The listing builds one solid part. Answer for the finished solid, in the listing's coordinates (mm). Round coordinates to 2 decimals unless told otherwise and drop trailing zeros. Write each loop counter-clockwise with the first axis right and the second up, starting at its lowest first coordinate (ties: lowest second). Pieces come first, ordered by that corner, then holes. Notation, with made-up numbers: (6.5, 74.25) - (23.5, 74.25) arc R23 ccw to (23.5, 95.25) - close; hole circle Ø7 at (59, 52.5). An arc over 180 degrees is marked (long way). Return JSON: item names as keys, results as strings. Group by question number.
(1) Section C-C, the plane x = -87 is taken. Write down the section's boundary in (y, z), then the cut area to 3 significant figures.
(2) Section B-B, the plane z = 1.1 is taken. Give the number of separate pieces and of enclosed holes in the cut face, then the cut area to 3 significant figures.
(3) Section A-A, the plane y = 2 is taken. Write down the section's boundary in (x, z).
(4) Find the intervals of material crossed by line 1 along X through (y, z) = (-32.5, 2.25); line 2 along X through (y, z) = (-71.5, 1.55); line 3 along X through (y, z) = (-113.5, 4.65), in increasing order. Write a range as [from, to].
(5) Each of these flat-tipped pins is pushed along its axis until it touches: pin 1 (1 mm diameter, centred on y = -82.5, z = 2, fed in from -X); pin 2 (6 mm diameter, centred on x = 94.92, y = -69.92, fed in from -Z); pin 3 (2.5 mm diameter, centred on y = -109, z = 2, fed in from +X). Where does it stop, or does it pass through?
```python
from build123d import *

# Parameters (mm, degrees)
F0_W      = 220
F0_H      = 170
F0_W_2    = 200
F0_H_2    = 150
F1_DEPTH  = 5
F2_W      = 5.5
F2_H      = 21
F3_DEPTH  = 25
F4_W      = 12
F4_H      = 5
F5_DEPTH  = 45
F6_R      = 2.2
F7_DEPTH  = 25
F8_R      = 5.99999
F9_R      = 6
F10_R     = 4
F11_DEPTH = 2.5
F13_R     = 5
F15_DEPTH = 3
F12_R     = 2.5
F16_DEPTH = 3


# Not quite as in the source:
# - a fillet or chamfer is up to 0.001 mm smaller than in the source, because OpenCascade refuses the exact size


with BuildPart() as f1:
    # F0 (on Top) → F1 (new body)
    with BuildSketch(Plane.XY):
        Rectangle(F0_W, F0_H)
        Rectangle(F0_W_2, F0_H_2, mode=Mode.SUBTRACT)
        Rectangle(F0_W_2, F0_H_2)
    extrude(amount=F1_DEPTH)

    # F2 (on face) → F3 (cut)
    with BuildSketch(Plane.XY.offset(5)):
        with Locations((-105, 60)):
            Rectangle(F2_W, F2_H)
        with Locations((-105, 10)):
            Rectangle(F2_W, F2_H)
        with Locations((-105, -40)):
            Rectangle(F2_W, F2_H)
        with Locations((105, 60)):
            Rectangle(F2_W, F2_H)
        with Locations((105, 10)):
            Rectangle(F2_W, F2_H)
        with Locations((105, -40)):
            Rectangle(F2_W, F2_H)
    extrude(amount=-F3_DEPTH, mode=Mode.SUBTRACT)

    # F4 (on face) → F5 (join)
    with BuildSketch(Plane.XZ.offset(85)):
        with Locations((59, 2.5)):
            Rectangle(F4_W, F4_H)
        with Locations((-59, 2.5)):
            Rectangle(F4_W, F4_H)
    extrude(amount=F5_DEPTH)

    # F6 (on face) → F7 (cut)
    with BuildSketch(Plane.XY.offset(5)):
        with Locations((-59, -74.3)):
            Circle(F6_R)
        with Locations((-59, -124)):
            Circle(F6_R)
        with Locations((59, -74.3)):
            Circle(F6_R)
        with Locations((59, -124)):
            Circle(F6_R)
    extrude(amount=-F7_DEPTH, mode=Mode.SUBTRACT)

    # F8 (radius 6 in the source; OpenCascade refuses exactly that, so slightly less here)
    f8_edges = [f1.edges().sort_by_distance(p)[0] for p in [
        (-65, -130, 2.5),
        (-53, -130, 2.5),
        (53, -130, 2.5),
        (65, -130, 2.5),
    ]]
    fillet(f8_edges, radius=F8_R)

    # F9
    f9_edges = [f1.edges().sort_by_distance(p)[0] for p in [
        (-65, -85, 2.5),
        (-53, -85, 2.5),
        (53, -85, 2.5),
        (65, -85, 2.5),
    ]]
    fillet(f9_edges, radius=F9_R)

    # F10 (on face) → F11 (cut)
    with BuildSketch(Plane.XY.offset(5)):
        with Locations((-59, -124)):
            Circle(F10_R)
        with Locations((-59, -74.3)):
            Circle(F10_R)
        with Locations((59, -74.3)):
            Circle(F10_R)
        with Locations((59, -124)):
            Circle(F10_R)
    extrude(amount=-F11_DEPTH, mode=Mode.SUBTRACT)

    # F13
    f13_edges = [f1.edges().sort_by_distance(p)[0] for p in [
        (-110, -85, 2.5),
        (110, -85, 2.5),
        (110, 85, 2.5),
        (-110, 85, 2.5),
    ]]
    fillet(f13_edges, radius=F13_R)

    # F14 (on face) → F15 (cut)
    with BuildSketch(Plane.XY):
        Polygon((-98.42, -67.8992740578), (-98.42, -71.9407259422), (-94.92, -73.9614518843), (-91.42, -71.9407259422), (-91.42, -67.8992740578), (-94.92, -65.8785481157), align=None)
        Polygon((98.42, -71.9407259422), (98.42, -67.8992740578), (94.92, -65.8785481157), (91.42, -67.8992740578), (91.42, -71.9407259422), (94.92, -73.9614518843), align=None)
    extrude(amount=F15_DEPTH, mode=Mode.SUBTRACT)

    # F12 (on face) → F16 (cut)
    with BuildSketch(Plane.XY.offset(5)):
        with Locations((94.92, -69.92)):
            Circle(F12_R)
        with Locations((-94.92, -69.92)):
            Circle(F12_R)
    extrude(amount=-F16_DEPTH, mode=Mode.SUBTRACT)


solid = f1.part
```
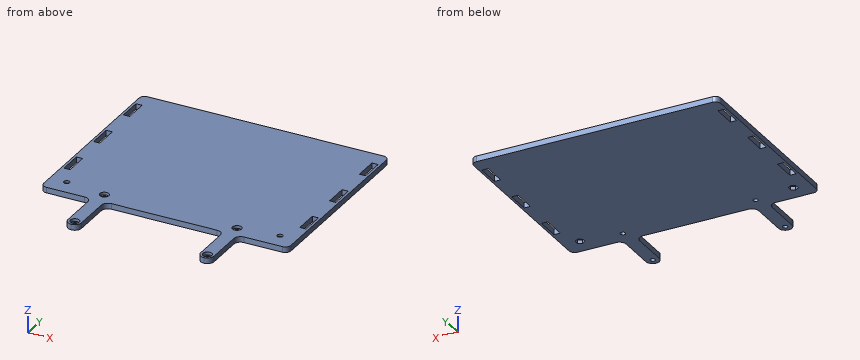
Working result:
{
 "1": {"outline": "(-85, 0) - (85, 0) - (85, 5) - (-85, 5) - close", "area": "850 mm^2"},
 "2": {"separate pieces": "1", "enclosed holes": "12", "area": "37,600 mm^2"},
 "3": {"outline": "(-110, 0) - (-107.75, 0) - (-107.75, 5) - (-110, 5) - close; (-102.25, 0) - (102.25, 0) - (102.25, 5) - (-102.25, 5) - close; (107.75, 0) - (110, 0) - (110, 5) - (107.75, 5) - close"},
 "4": {"line 1": "x = [-110, -107.75], [-102.25, 102.25], [107.75, 110]", "line 2": "x = [-110, -98.42], [-91.42, 91.42], [98.42, 110]", "line 3": "x = [-65, -53], [53, 65]"},
 "5": {"pin 1": "stops at x = -109.58", "pin 2": "stops at z = 3", "pin 3": "stops at x = 65"}
}
